Source: CAD feature listing. Evaluate the final solid. Frame: model axes, mm. A direction names the side the tool comes from. Round coordinates to 2 decimals unless told otherwise and drop trailing zeros. Write each loop counter-clockwise with the first axis right and the second up, starting at its lowest first coordinate (ties: lowest second). Pieces come first, ordered by that corner, then holes.
from build123d import *

# Parameters (mm, degrees)
SKETCH1_R               = 25.4
EXTRUDE1_DEPTH          = 50.8
SKETCH2_R               = 12.7
EXTRUDE2_DEPTH          = 495.3
SKETCH3_R               = 6.35
CUT_EXTRUDE1_DEPTH      = 26.4
CUT_EXTRUDE1_DEPTH_BACK = 26.4


with BuildPart() as part:
    # Sketch1 → Extrude1 (new body)
    with BuildSketch(Plane.XY):
        Circle(SKETCH1_R)
    extrude(amount=EXTRUDE1_DEPTH)

    # Sketch2 → Extrude2 (add)
    with BuildSketch(Plane.XY.offset(50.8)):
        Circle(SKETCH2_R)
    extrude(amount=EXTRUDE2_DEPTH)

    # Sketch3 → Cut-Extrude1 (cut, two sides)
    with BuildSketch(Plane(origin=(0, 0, 0), x_dir=(0, 0, -1), z_dir=(1, 0, 0))) as cut_extrude1_sk:
        with Locations((-27.347285404, 0)):
            Circle(SKETCH3_R)
    extrude(amount=CUT_EXTRUDE1_DEPTH, mode=Mode.SUBTRACT)
    extrude(cut_extrude1_sk.sketch, amount=-CUT_EXTRUDE1_DEPTH_BACK, mode=Mode.SUBTRACT)


solid = part.part
1) Contact query for flat-ended pins moving along their axis: P1, Ø10, axis at x = 9, y = 16, coming from the +Z side; P2, Ø11.5, axis at y = 0, z = 27.35, coming from the +X side; P3, Ø4, axis at x = 13, z = 141, coming from the -Y side; P4, Ø3, axis at x = -9.5, y = 12.5, coming from the -Z side. Output: stop coordinate, or through.
Taken from the geometry:
P1: stops at z = 50.8
P2: passes through
P3: stops at y = -6.35
P4: stops at z = 0
2) Material intervals for line 1 (Z direction, x = 11.5, y = 1); line 2 (Z direction, x = -9.25, y = 0); line 3 (Z direction, x = -17, y = 16), sorted ascending.
Taken from the geometry:
line 1: z = 0 to 21.08, 33.62 to 546.1
line 2: z = 0 to 21, 33.7 to 546.1
line 3: z = 0 to 50.8
3) Section query C-C on z = 159. Return the cut outline in (x, y).
Taken from the geometry:
outline: circle Ø25.4 at (0, 0)
4) Section query B-B on x = -18.5. Return the cut outline in (y, z).
Taken from the geometry:
outline: (-17.4, 0) - (17.4, 0) - (17.4, 50.8) - (-17.4, 50.8) - close; hole circle Ø12.7 at (0, 27.35)
5) Section query A-A on y = 0. Return the cut outline in (x, z), then the cut area to 3 significant figures.
Taken from the geometry:
outline: (-25.4, 0) - (25.4, 0) - (25.4, 21) - (-25.4, 21) - close; (-25.4, 33.7) - (25.4, 33.7) - (25.4, 50.8) - (12.7, 50.8) - (12.7, 546.1) - (-12.7, 546.1) - (-12.7, 50.8) - (-25.4, 50.8) - close
area: 14,500 mm2
6) Reachability of faces 1 (the face through (-2.75, -12.4, 294.98)), 2 (the face through (24.227, 7.629, 25.044)) from +Z, -Z, +X, -X, +Y, -Y: full face, straight path, thin tool, end or side. Return the list, or none.
Taken from the geometry:
face 1: +Z
face 2: +Z, -Z
